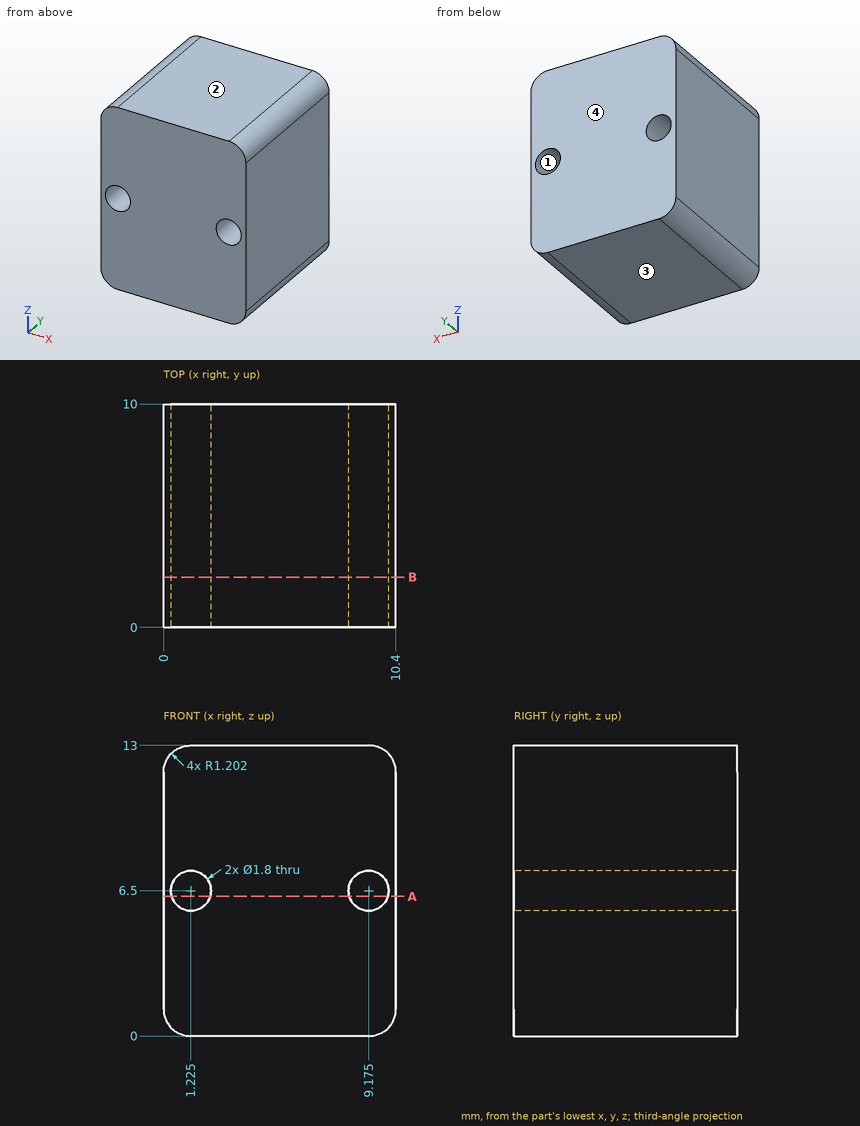
For this review, use the dimensioned drawing (mm, ordinates from the lowest corner) and the shaded views. Give positions to 0.01 mm unless a question says otherwise; leave off trailing zeros. Loops run counter-clockwise (first coordinate to the right, second up) from the corner with the lowest first, then second, coordinate; pieces in that order, holes last. Notation, with made-up numbers: (-37.75, 86) -> (-21.75, 86) arc R38 cw to (-21.75, 125) -> close; hole circle Ø3 at (39, 7). An arc over 180 degrees is marked (long way). One line per question, with ' | ' between items. Start each with the question number.
(1) We need section B-B (y = 2.25). State the section outline as (x, z) points (3 decimals), and give its area (3 significant figures).
(2) Insertion check: P1, Ø1.1, axis at x = 9.175, z = 6.5, coming from the +Y side. The pin has a flat end and moves straight along its axis. Give the tip position at first contact, or say it passes through.
(3) We need section A-A (z = 6.25). State the section outline as (x, y) points, and give its area (3 significant figures).
(4) For line 1 (X direction, y = 5.5, z = 6.5) (3 decimals); line 2 (Z direction, x = 2, y = 5); line 3 (Z direction, x = 8.5, y = 4.5), list the stretches that pass through material, from the lowest coordinate up.
(5) Draft analysis for pull direction Z (two halves, no side actions). For the marked faces 1, 2, 3 and 4, state which applies: +Z half, -Z half, draft (parallel to the pull), parting line (faces both ways), or undercut.
The answers:
1) outline: (0, 1.202) arc R1.202 ccw to (1.202, 0) -> (9.198, 0) arc R1.202 ccw to (10.4, 1.202) -> (10.4, 11.798) arc R1.202 ccw to (9.198, 13) -> (1.202, 13) arc R1.202 ccw to (0, 11.798) -> close; hole circle Ø1.8 at (1.225, 6.5); hole circle Ø1.8 at (9.175, 6.5) | area: 129 mm^2
2) P1: passes through
3) outline: (0, 0) -> (0.36, 0) -> (0.36, 10) -> (0, 10) -> close; (2.09, 0) -> (8.31, 0) -> (8.31, 10) -> (2.09, 10) -> close; (10.04, 0) -> (10.4, 0) -> (10.4, 10) -> (10.04, 10) -> close | area: 69.4 mm^2
4) line 1: x = 0 to 0.325, 2.125 to 8.275, 10.075 to 10.4 | line 2: z = 0 to 6.04, 6.96 to 13 | line 3: z = 0 to 5.9, 7.1 to 13
5) face 1: undercut | face 2: +Z half | face 3: -Z half | face 4: draft
